Answer from the drawing. Dimensions are ordinates in mm from the lowest x, y and z of the part. A direction names the side the tool comes from. Round coordinates to 2 decimals unless told otherwise and drop trailing zeros. Order: outer loops, then holes, each group sorted by start corner. A loop starts at its lowest first (then second) coordinate and runs counter-clockwise, first axis right, second up. Notation, with made-up numbers: M 58.5,37.5 L 92.5,37.5 A21 cw 92.5,75.5 Z; hole C 44.25,47.25 d11. An arc over 180 degrees is marked long. Use one line per item in the form item = value. Start each with the question number.
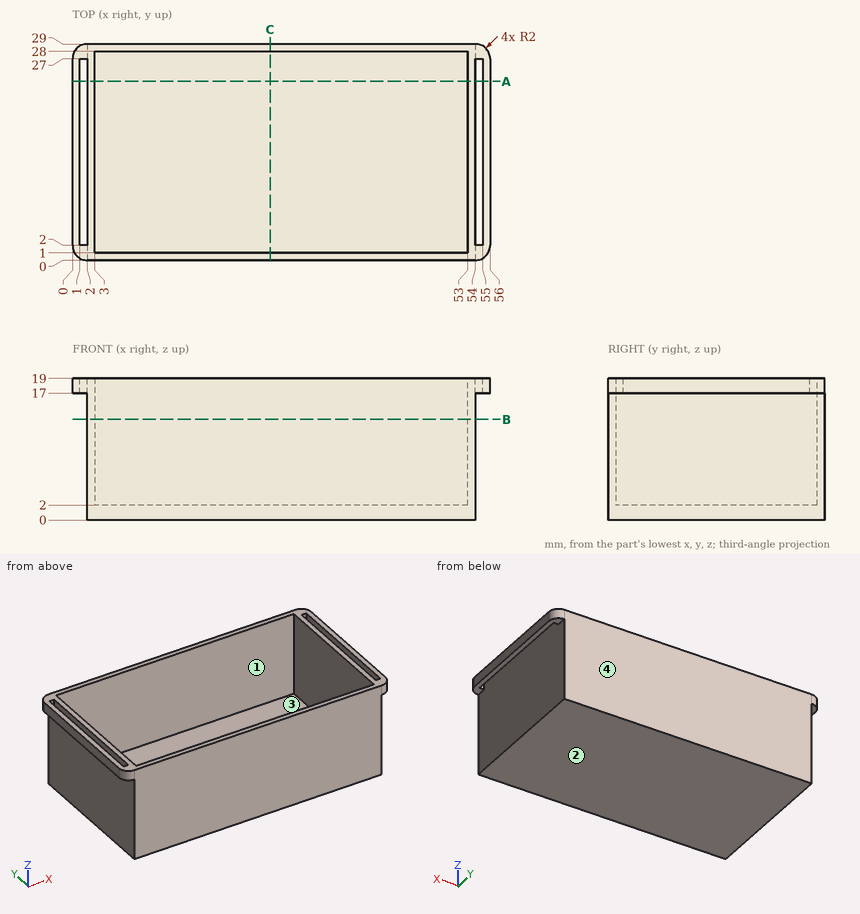
Item 1: Section B-B (z = 13.5) is taken. Write down the section's boundary in (x, y).
Item 2: Given P1, Ø1.1, axis at x = 54.5, z = 18, coming from the -Y side; P2, Ø9.5, axis at y = 8, z = 5.5, coming from the -X side; P3, Ø0.6, axis at x = 0.5, y = 10, coming from the -Z side; P4, Ø1.5, axis at y = 11, z = 3, coming from the +X side, each flat-ended and moving along its own axis, determine where each tip first touches the part or whether it passes through.
Item 3: A tool of negligible diameter and unlimited length cuts with its end or side. For the marked faces 3 and 4, from which of +Z, -Z, +X, -X, +Y, -Y can it reach the whole face along a straight path? Write none if from no direction.
Item 4: Section C-C (x = 26.5) is taken. Write down the section's boundary in (y, z), and give its area (3 significant figures).
Item 5: Find the intervals of material crossed by L1, parallel to Y at x = 32.5, z = 3.5; L2, parallel to X at y = 9.75, z = 7.5; L3, parallel to Z at x = 44, y = 24.25, in increasing order. Write a range as [from, to].
Item 6: For a pull along X with two mould halves and no side action, classify the marked faces 1 and 2 as pulls with the +X half, pulls with the -X half, needs draft (parallel to the pull), parting line crosses it, or undercut.
Item 7: Section A-A (y = 24) is taken. Write down the section's boundary in (x, z).
The answers:
q1.outline = M 2,0 L 54,0 L 54,29 L 2,29 Z; hole M 3,1 L 53,1 L 53,28 L 3,28 Z
q2.P1 = 0
q2.P2 = 2
q2.P3 = 17
q2.P4 = 54
q3.face_3 = +Z
q3.face_4 = +Z, -Z, +X, -X, +Y
q4.outline = M 0,0 L 29,0 L 29,19 L 28,19 L 28,2 L 1,2 L 1,19 L 0,19 Z
q4.area = 92.0 mm²
q5.L1 = [0, 1], [28, 29]
q5.L2 = [2, 3], [53, 54]
q5.L3 = [0, 2]
q6.face_1 = undercut
q6.face_2 = needs draft
q7.outline = M 0,17 L 1,17 L 1,19 L 0,19 Z; M 2,0 L 54,0 L 54,19 L 53,19 L 53,2 L 3,2 L 3,19 L 2,19 Z; M 55,17 L 56,17 L 56,19 L 55,19 Z
